Model file for the job. Use its own axes, mm. Face numbers are marked on the shaded views. Coordinates: 2 decimals unless noted, no trailing zeros. Loops run counter-clockwise (first coordinate to the right, second up) from the corner with the lowest first, then second, coordinate; pieces in that order, holes last.
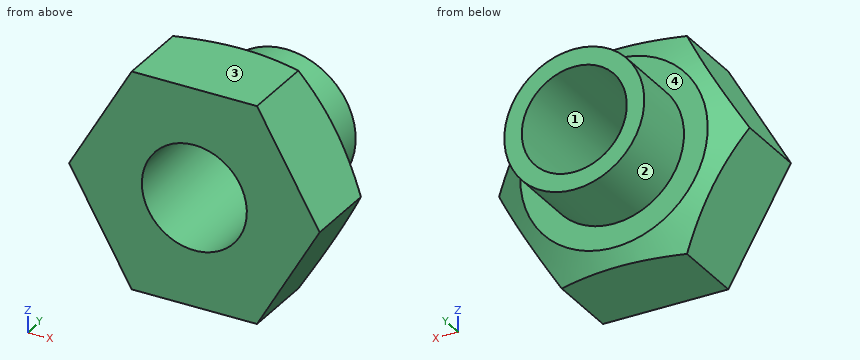
from build123d import *

# Parameters (mm, degrees)
BOSS_EXTRUDE1_DEPTH = 65
SKETCH7_R           = 50
BOSS_EXTRUDE2_DEPTH = 50
SKETCH8_R           = 37.5
CUT_EXTRUDE1_DEPTH  = 166.044186003


with BuildPart() as part:
    # Sketch1 → Boss-Extrude1 (new body)
    with BuildSketch(Plane(origin=(0, 0, 0), x_dir=(1, 0, 0), z_dir=(0, 1, 0))):
        Polygon((44.744645862, -77.5), (89.489291724, 0), (44.744645862, 77.5), (-44.744645862, 77.5), (-89.489291724, 0), (-44.744645862, -77.5), align=None)
    extrude(amount=BOSS_EXTRUDE1_DEPTH)

    # Sketch5 → Cut-Revolve1 (revolve, cut)
    with BuildSketch(Plane.XY, mode=Mode.PRIVATE) as cut_revolve1_sk:
        Polygon((66.946176196, 65), (89.489291724, 65), (89.489291724, 51.984726181), align=None)
    revolve(cut_revolve1_sk.sketch.rotate(Axis((0, 80.544335103, 0), (0, -1, 0)), 300.000000001), axis=Axis((0, 80.544335103, 0), (0, -1, 0)), mode=Mode.SUBTRACT)

    # Sketch7 → Boss-Extrude2 (add)
    with BuildSketch(Plane(origin=(0, 65, 0), x_dir=(1, 0, 0), z_dir=(0, 1, 0))):
        with Locations(Location((0, 0, 0), (0, 0, 270))):
            Circle(SKETCH7_R)
    extrude(amount=BOSS_EXTRUDE2_DEPTH)

    # Sketch8 → Cut-Extrude1 (cut, through all)
    with BuildSketch(Plane(origin=(0, 115, 0), x_dir=(1, 0, 0), z_dir=(0, 1, 0))):
        with Locations(Location((0, 0, 0), (0, 0, 270))):
            Circle(SKETCH8_R)
    extrude(amount=-CUT_EXTRUDE1_DEPTH, mode=Mode.SUBTRACT)


solid = part.part
Q1. Flat gauge pins, fed straight in: P1, Ø4, axis at x = -32, z = 52.5, coming from the +Y side; P2, Ø6, axis at y = 26.5, z = -4.5, coming from the +X side; P3, Ø12, axis at x = -9.5, y = 74, coming from the +Z side. Where does each tip first touch, or does it go through?
Answers:
P1: stops at y = 65
P2: stops at x = 88.62
P3: stops at z = 49.88
Q2. Slice it at A-A (y = 25.5). List the corners of the cut face in (x, z).
Answers:
outline: (-89.49, 0) - (-44.74, -77.5) - (44.74, -77.5) - (89.49, 0) - (44.74, 77.5) - (-44.74, 77.5) - close; hole circle Ø75 at (0, 0)
Q3. Slice it at C-C (y = 69). List the corners of the cut face in (x, z).
Answers:
outline: circle Ø100 at (0, 0); hole circle Ø75 at (0, 0)
Q4. Drill centre lines: line 1 (Y direction, x = -53, z = -28.5); line 2 (X direction, y = 110, z = -3.5); line 3 (Z direction, x = 29.5, y = 108.5). Where is each one in solid material? Low to high.
Answers:
line 1: y = 0 to 65
line 2: x = -49.88 to -37.34, 37.34 to 49.88
line 3: z = -40.37 to -23.15, 23.15 to 40.37
Q5. Mould opens along Z. For the marked faces 1, 2, 3 and 4 say: +Z half, -Z half, draft (parallel to the pull), parting line (faces both ways), or undercut.
Answers:
face 1: undercut
face 2: parting line
face 3: +Z half
face 4: draft
Q6. Slice it at B-B (x = 0). List the corners of the cut face in (y, z), and give its area (3 significant figures).
Answers:
outline: (0, -77.5) - (58.91, -77.5) - (65, -66.95) - (65, -50) - (115, -50) - (115, -37.5) - (0, -37.5) - close; (0, 37.5) - (115, 37.5) - (115, 50) - (65, 50) - (65, 66.95) - (58.91, 77.5) - (0, 77.5) - close
area: 6,390 mm2
